Verification items for the finished model (mm, model axes). Face numbers are marked on the shaded views. Give positions to 0.01 mm unless a question says otherwise; leave off trailing zeros. Order: outer loops, then holes, each group sorted by start corner. A loop starts at its lowest first (then second) coordinate and runs counter-clockwise, first axis right, second up. Notation, with made-up numbers: (-3, 55.25) - (50, 55.25) arc R18 cw to (50, 62.25) - close; hole circle Ø8 at (35, 18). An arc over 180 degrees is marked (long way). Answer as a JSON object with one key per item and string values.
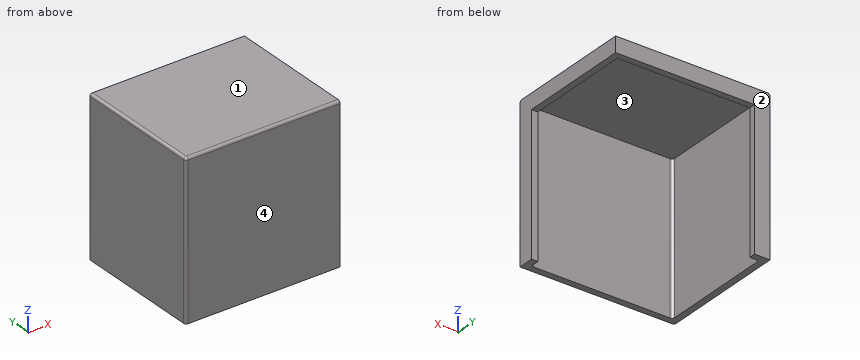
```python
from build123d import *

# Parameters (mm, degrees)
F1_DEPTH = 2.5
F2_DEPTH = 57.5
F3_DEPTH = 3.5
F4_R     = 1


with BuildPart() as f1:
    # F0 (on Top) → F1 (new body)
    with BuildSketch(Plane.XY):
        Polygon((26.914498, 24.649286), (-24.585502, 24.649286), (-28.085502, 24.649286), (-28.085502, -20.350714), (26.914498, -20.350714), (26.914498, -16.850714), align=None)
        Polygon((-24.585502, 27.149286), (-30.585502, 27.149286), (-30.585502, -22.850714), (29.414498, -22.850714), (29.414498, -16.850714), (26.914498, -16.850714), (26.914498, -20.350714), (-28.085502, -20.350714), (-28.085502, 24.649286), (-24.585502, 24.649286), align=None)
        Polygon((29.414498, 27.149286), (-24.585502, 27.149286), (-24.585502, 24.649286), (26.914498, 24.649286), (26.914498, -16.850714), (29.414498, -16.850714), align=None)
    extrude(amount=F1_DEPTH)

    # F0 (on Top) → F2 (join)
    with BuildSketch(Plane.XY):
        Polygon((-24.585502, 27.149286), (-30.585502, 27.149286), (-30.585502, -22.850714), (29.414498, -22.850714), (29.414498, -16.850714), (26.914498, -16.850714), (26.914498, -20.350714), (-28.085502, -20.350714), (-28.085502, 24.649286), (-24.585502, 24.649286), align=None)
    extrude(amount=-F2_DEPTH)

    # F0 (on Top) → F3 (join)
    with BuildSketch(Plane.XY):
        Polygon((29.414498, 27.149286), (-24.585502, 27.149286), (-24.585502, 24.649286), (26.914498, 24.649286), (26.914498, -16.850714), (29.414498, -16.850714), align=None)
    extrude(amount=-F3_DEPTH)

    # F4
    f4_edges = [f1.edges().sort_by_distance(p)[0] for p in [
        (-30.585502, 2.149286, 2.5),
        (-0.585502, -22.850714, 2.5),
        (-30.585502, -22.850714, -27.5),
        (-28.085502, -20.350714, -28.75),
        (26.914498, -20.350714, -28.75),
        (-28.085502, 24.649286, -28.75),
    ]]
    fillet(f4_edges, radius=F4_R)


solid = f1.part
```
(1) Release check for a two-part mould opening along Y. For the marked faces 1, 2, 3 and 4 record: pulls with the +Y half, pulls with the -Y half, needs draft (parallel to the pull), parting line crosses it, or undercut.
Computed values:
{"face 1": "needs draft", "face 2": "pulls with the +Y half", "face 3": "undercut", "face 4": "pulls with the -Y half"}
(2) Section check B-B (z = -28). Record the cut outline in (x, y), then the cut area to 3 significant figures.
Computed values:
{"outline": "(-30.59, -21.85) arc R1 ccw to (-29.59, -22.85) - (29.41, -22.85) - (29.41, -16.85) - (26.91, -16.85) - (26.91, -19.35) arc R1 cw to (25.91, -20.35) - (-27.09, -20.35) arc R1 cw to (-28.09, -19.35) - (-28.09, 23.65) arc R1 cw to (-27.09, 24.65) - (-24.59, 24.65) - (-24.59, 27.15) - (-30.59, 27.15) - close", "area": "287 mm²"}
(3) Section check A-A (y = 7). Record the cut outline in (x, z), then the cut area to 3 significant figures.
Computed values:
{"outline": "(-30.59, -57.5) - (-28.09, -57.5) - (-28.09, 0) - (26.91, 0) - (26.91, -3.5) - (29.41, -3.5) - (29.41, 2.5) - (-29.59, 2.5) arc R1 ccw to (-30.59, 1.5) - close", "area": "302 mm²"}
(4) Gauge pin test, flat ends, axial feed: pin 1 Ø2 at (y, z) = (14, -37.5) entering from +X; pin 2 Ø2 at (y, z) = (26.5, -38) entering from +X; pin 3 Ø22 at (x, y) = (4, 4.5) entering from -Z. Record the tip position at first contact, or that the pin passes through.
Computed values:
{"pin 1": "stops at x = -28.09", "pin 2": "stops at x = -24.59", "pin 3": "stops at z = 0"}
(5) Material ranges on line 1 along Y through (x, z) = (11.5, -1); line 2 along Z through (x, y) = (-10, 4.5); line 3 along X through (y, z) = (18, -13.5), recorded low to high. Write a range as [from, to].
Computed values:
{"line 1": "y = [-22.85, -20.35], [24.65, 27.15]", "line 2": "z = [0, 2.5]", "line 3": "x = [-30.59, -28.09]"}
(6) Section check C-C (x = -1). Record the cut outline in (y, z), then the cut area to 3 significant figures.
Computed values:
{"outline": "(-22.85, -57.5) - (-20.35, -57.5) - (-20.35, 0) - (24.65, 0) - (24.65, -3.5) - (27.15, -3.5) - (27.15, 2.5) - (-21.85, 2.5) arc R1 ccw to (-22.85, 1.5) - close", "area": "277 mm²"}
